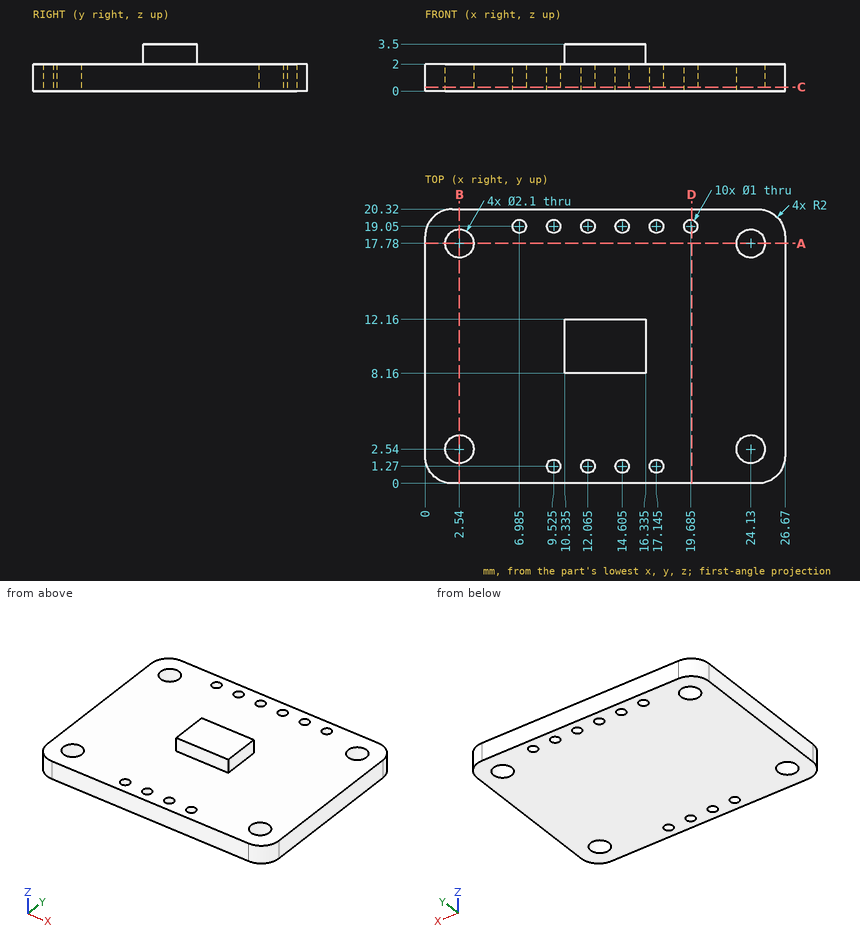
Study the drawing (mm; zero at the part's minimum x, y, z) and answer. Round coordinates to 2 decimals unless told otherwise and drop trailing zeros. Write each loop counter-clockwise with the first axis right and the second up, starting at its lowest first coordinate (ties: lowest second). Pieces come first, ordered by that corner, then holes. Notation, with made-up numbers: (5.25, 49.25) - (58.25, 49.25) arc R17 cw to (58.25, 53.25) - close; hole circle Ø4 at (-15, 3). An arc over 180 degrees is marked (long way). Return JSON: item names as keys, results as strings. Group by question number.
Q1. The part is cut by section C-C on z = 0.3. Count the separate pieces of the cut face and the enclosed holes in it, then the cut area to 3 significant figures.
Q2. The part is cut by section D-D on x = 19.75. Write down the section's boundary in (y, z).
Q3. The part is cut by section B-B on x = 2.54. Write down the section's boundary in (y, z), then the cut area to 3 significant figures.
Q4. Find the intervals of material crossed by L1, parallel to Y at x = 2.54, z = 1.5; L2, parallel to Y at x = 14.25, z = 1.9; L3, parallel to X at y = 3.25, z = 1.05, in increasing order.
Q5. Each of these flat-tipped pins is pushed along its axis until it touches: pin 1 Ø2 at (x, y) = (8, 2.5) entering from +Z; pin 2 Ø3.5 at (x, y) = (24.13, 2.54) entering from -Z; pin 3 Ø1.6 at (y, z) = (10.5, 3) entering from +X (3 decimals); pin 4 Ø1.3 at (x, y) = (24.13, 17.78) entering from -Z. Where does it stop, or does it pass through?
Q6. The part is cut by section A-A on y = 17.78. Write down the section's boundary in (x, z), then the cut area to 3 significant figures.
Solved:
{
 "1": {"separate pieces": "1", "enclosed holes": "14", "area": "517 mm²"},
 "2": {"outline": "(0, 0) - (18.55, 0) - (18.55, 2) - (0, 2) - close; (19.55, 0) - (20.32, 0) - (20.32, 2) - (19.55, 2) - close"},
 "3": {"outline": "(0, 0) - (1.49, 0) - (1.49, 2) - (0, 2) - close; (3.59, 0) - (16.73, 0) - (16.73, 2) - (3.59, 2) - close; (18.83, 0) - (20.32, 0) - (20.32, 2) - (18.83, 2) - close", "area": "32.2 mm²"},
 "4": {"L1": "0 to 1.49, 3.59 to 16.73, 18.83 to 20.32", "L2": "0 to 0.92, 1.62 to 18.7, 19.4 to 20.32", "L3": "0 to 1.77, 3.31 to 23.36, 24.9 to 26.67"},
 "5": {"pin 1": "z = 2", "pin 2": "z = 0", "pin 3": "x = 16.335", "pin 4": "through"},
 "6": {"outline": "(0, 0) - (1.49, 0) - (1.49, 2) - (0, 2) - close; (3.59, 0) - (23.08, 0) - (23.08, 2) - (3.59, 2) - close; (25.18, 0) - (26.67, 0) - (26.67, 2) - (25.18, 2) - close", "area": "44.9 mm²"}
}
